```python
from build123d import *

# Parameters (mm, degrees)
SKETCH1_W                       = 80
SKETCH1_H                       = 40
SKETCH1_R                       = 7
SKETCH1_R_2                     = 3
BOSS_EXTRUDE1_DEPTH             = 8
CUT_EXTRUDE1_OUTLINE_R          = 7
CUT_EXTRUDE1_OUTLINE_R_2        = 3
CUT_EXTRUDE1_DEPTH              = 4.5
FILLET1_R                       = 5
CBORE_FOR_M3_SHCS1_AT_2_COUNT   = 2
CBORE_FOR_M3_SHCS1_AT_2_PITCH   = 52
M4X0_7_TAPPED_HOLE4_D           = 3.3
M4X0_7_TAPPED_HOLE4_DEPTH       = 40
M4X0_7_TAPPED_HOLE4_CSINK_D     = 4.05
M4X0_7_TAPPED_HOLE4_CSINK_ANGLE = 90
M4X0_7_TAPPED_HOLE4_TIP         = 0.991420021
CHAMFER1_SIZE                   = 0.75


# Read off the part's stored shape, not the designer's step: Cut-Extrude1
with BuildPart() as part:
    # Sketch1 → Boss-Extrude1 (new body)
    # profile 1 of 3: a face of its own
    with BuildSketch(Plane.XY):
        Rectangle(SKETCH1_W, SKETCH1_H)
        with Locations((15, 0)):
            Circle(SKETCH1_R, mode=Mode.SUBTRACT)
        with Locations((-15, 0)):
            Circle(SKETCH1_R, mode=Mode.SUBTRACT)
    # profile 2 of 3: a face of its own
    with BuildSketch(Plane.XY):
        with Locations((15, 0)):
            Circle(SKETCH1_R)
        with Locations((15, 0)):
            Circle(SKETCH1_R_2, mode=Mode.SUBTRACT)
    # profile 3 of 3: a face of its own
    with BuildSketch(Plane.XY):
        with Locations((-15, 0)):
            Circle(SKETCH1_R)
        with Locations((-15, 0)):
            Circle(SKETCH1_R_2, mode=Mode.SUBTRACT)
    extrude(amount=BOSS_EXTRUDE1_DEPTH)

    # Cut-Extrude1 outline → Cut-Extrude1 (cut)
    # profile 1 of 2: a face of its own
    with BuildSketch(Plane.XY):
        with Locations((15, 0)):
            Circle(CUT_EXTRUDE1_OUTLINE_R)
        with Locations((15, 0)):
            Circle(CUT_EXTRUDE1_OUTLINE_R_2, mode=Mode.SUBTRACT)
    # profile 2 of 2: a face of its own
    with BuildSketch(Plane.XY):
        with Locations((-15, 0)):
            Circle(CUT_EXTRUDE1_OUTLINE_R)
        with Locations((-15, 0)):
            Circle(CUT_EXTRUDE1_OUTLINE_R_2, mode=Mode.SUBTRACT)
    extrude(amount=CUT_EXTRUDE1_DEPTH, mode=Mode.SUBTRACT)

    # Fillet1
    fillet1_edges = [part.edges().sort_by_distance(p)[0] for p in [
        (40, -20, 4),
        (-40, -20, 4),
        (-40, 20, 4),
        (40, 20, 4),
    ]]
    fillet(fillet1_edges, radius=FILLET1_R)

    # Sketch2 → CBORE for M3 SHCS1 (revolve, cut)
    with BuildSketch(Plane(origin=(26, -10, 0), x_dir=(0, 1, 0), z_dir=(1, 0, 0))):
        Polygon((0, 0), (0, 8), (1.7, 8), (1.7, 3), (3.25, 3), (3.25, 0.025), (3.275, 0), align=None)
    cbore_for_m3_shcs1 = revolve(axis=Axis((26, -10, -6.35), (0, 0, 1)), mode=Mode.SUBTRACT)

    # CBORE for M3 SHCS1 at 2: CBORE for M3 SHCS1 ×2
    with Locations(*[(-i * CBORE_FOR_M3_SHCS1_AT_2_PITCH, 0, 0) for i in range(1, CBORE_FOR_M3_SHCS1_AT_2_COUNT)]):
        add(cbore_for_m3_shcs1, mode=Mode.SUBTRACT)

    # M4x0.7 Tapped Hole4
    with Locations(Plane(origin=(0, -20, 0), x_dir=(-1, 0, 0), z_dir=(0, -1, 0))):
        with Locations((0, -4), (30, -4), (-30, -4)):
            CounterSinkHole(M4X0_7_TAPPED_HOLE4_D / 2, M4X0_7_TAPPED_HOLE4_CSINK_D / 2, depth=M4X0_7_TAPPED_HOLE4_DEPTH, counter_sink_angle=M4X0_7_TAPPED_HOLE4_CSINK_ANGLE)
            with Locations((0, 0, -(M4X0_7_TAPPED_HOLE4_DEPTH + M4X0_7_TAPPED_HOLE4_TIP / 2))):  # 118° drill point
                Cone(0, M4X0_7_TAPPED_HOLE4_D / 2, M4X0_7_TAPPED_HOLE4_TIP, mode=Mode.SUBTRACT)

    # Sketch8 → Tap Drill for M4x0.7 Tap1 (revolve, cut)
    with BuildSketch(Plane(origin=(-40, -12, 4), x_dir=(0, 0, 1), z_dir=(0, 1, 0))):
        Polygon((0, 0), (0, 12.991420021), (1.65, 12), (1.65, 0.025), (1.675, 0), align=None)
    tap_drill_for_m4x0_7_tap1 = revolve(axis=Axis((-46.35, -12, 4), (1, 0, 0)), mode=Mode.SUBTRACT)

    # Mirror1: Tap Drill for M4x0.7 Tap1 across plane
    add(tap_drill_for_m4x0_7_tap1.mirror(Plane(origin=(0, 0, 0), x_dir=(0, 0, 1), z_dir=(1, 0, 0))), mode=Mode.SUBTRACT)

    # Chamfer1
    chamfer1_edges = [part.edges().sort_by_distance(p)[0] for p in [
        (-22, 0, 0),
        (-18, 0, 8),
        (8, 0, 0),
        (12, 0, 8),
        (40, 0, 0),
        (40, 0, 8),
        (0, -20, 0),
        (-40, 0, 0),
        (0, 20, 0),
        (38.535533906, 18.535533906, 0),
        (-38.535533906, 18.535533906, 0),
        (-38.535533906, -18.535533906, 0),
        (38.535533906, -18.535533906, 0),
        (0, -20, 8),
        (0, 20, 8),
        (-40, 0, 8),
        (38.535533906, 18.535533906, 8),
        (-38.535533906, 18.535533906, 8),
        (-38.535533906, -18.535533906, 8),
        (38.535533906, -18.535533906, 8),
    ]]
    chamfer(chamfer1_edges, length=CHAMFER1_SIZE)


solid = part.part
```
The listing builds one solid part. Answer for the finished solid, in the listing's coordinates (mm). A direction names the side the tool comes from. Round coordinates to 2 decimals unless told otherwise and drop trailing zeros. Write each loop counter-clockwise with the first axis right and the second up, starting at its lowest first coordinate (ties: lowest second). Pieces come first, ordered by that corner, then holes. Notation, with made-up numbers: (6.25, 42.25) -> (10.25, 42.25) arc R19 cw to (10.25, 58.25) -> close; hole circle Ø7 at (37, 32). An arc over 180 degrees is marked (long way). Write item = value, one per line.
1) Given pin 1 (4 mm diameter, centred on x = 15, y = 3, fed in from -Z); pin 2 (3 mm diameter, centred on x = -27, y = -10, fed in from -Z), each flat-ended and moving along its own axis, determine where each tip first touches the part or whether it passes through.
Check values:
pin_1 = 4.5
pin_2 = 3
2) For a pull along X with two mould halves and no side action, classify faces 1 (the cylindrical face through (-31.216, -16.606, 2.885)), 2 (the flat face through (-0.5, -20, 1.8)), 3 (the conical face through (-38.13, -18.06, 7.87)) as released by +X, released by -X, zero draft, split by the parting line, or undercut.
Check values:
face_1 = undercut
face_2 = zero draft
face_3 = released by -X
3) Section D-D on y = 1.5 is taken. Give the number of separate pieces and of enclosed holes in the cut face, plus the area to 3 significant figures.
Check values:
separate_pieces = 3
enclosed_holes = 3
area = 451 mm²
4) Section B-B on y = 13 is taken. Write down the section's boundary in (x, z).
Check values:
outline = (-40, 0.75) -> (-39.25, 0) -> (39.25, 0) -> (40, 0.75) -> (40, 7.25) -> (39.25, 8) -> (-39.25, 8) -> (-40, 7.25) -> close; hole circle Ø3.3 at (-30, 4); hole circle Ø3.3 at (0, 4); hole circle Ø3.3 at (30, 4)
5) Section A-A on x = 15 is taken. Write down the section's boundary in (y, z).
Check values:
outline = (-20, 0.75) -> (-19.25, 0) -> (-7.75, 0) -> (-7, 0.75) -> (-7, 4.5) -> (-3, 4.5) -> (-3, 7.25) -> (-3.75, 8) -> (-19.25, 8) -> (-20, 7.25) -> close; (3, 4.5) -> (7, 4.5) -> (7, 0.75) -> (7.75, 0) -> (19.25, 0) -> (20, 0.75) -> (20, 7.25) -> (19.25, 8) -> (3.75, 8) -> (3, 7.25) -> close
6) Section C-C on x = 0 is taken. Write down the section's boundary in (y, z) (3 decimals), plus the area to 3 significant figures.
Check values:
outline = (-20, 0.75) -> (-19.25, 0) -> (19.25, 0) -> (20, 0.75) -> (20, 2.35) -> (-19.625, 2.35) -> (-20, 1.975) -> close; (-20, 6.025) -> (-19.625, 5.65) -> (20, 5.65) -> (20, 7.25) -> (19.25, 8) -> (-19.25, 8) -> (-20, 7.25) -> close
area = 187 mm²
7) Straight lines are drawn through the part: line 1 along Z through (x, y) = (30, -14.25); line 2 along X through (y, z) = (-11, 6.25); line 3 along Y through (x, z) = (33, 4). For each, find the intervals that lie inside material, in ascending order. Write a range as [from, to].
Check values:
line_1 = [0, 2.35], [5.65, 8]
line_2 = [-40, -27.37], [-24.63, 24.63], [27.37, 40]
line_3 = [-20, -13.65], [-10.35, 20]
8) Which of the six approach directions +Z, -Z, +X, -X, +Y, -Y give full straight-line access (tool end or side, diameter ignored) to faces 4 (the cylindrical face through (38, -19, 4)), 5 (the cylindrical face through (8, 0, 3))?
Check values:
face_4 = +Z, -Z, +X, -Y
face_5 = -Z
